```python
from build123d import *

# Parameters (mm, degrees)
SKETCH1_R           = 2
SKETCH1_R_2         = 6.5
BOSS_EXTRUDE1_DEPTH = 6


with BuildPart() as part:
    # Sketch1 → Boss-Extrude1 (new body)
    with BuildSketch(Plane(origin=(0, 0, 0), x_dir=(1, 0, 0), z_dir=(0, 1, 0))):
        with BuildLine():
            Line((-22.107690969, 10.5), (-42.5, 10.5))
            ThreePointArc((-42.5, 10.5), (-53, 0), (-42.5, -10.5))
            Line((-42.5, -10.5), (-22.107690969, -10.5))
            ThreePointArc((-22.107690969, -10.5), (-19.800295422, -11.06424462), (-18.013674085, -12.629629684))
            ThreePointArc((-18.013674085, -12.629629684), (7.2e-08, -22), (18.013674168, -12.629629566))
            ThreePointArc((18.013674168, -12.629629566), (19.800295486, -11.064244587), (22.107690969, -10.5))
            Line((22.107690969, -10.5), (42.5, -10.5))
            ThreePointArc((42.5, -10.5), (53, 0), (42.5, 10.5))
            Line((42.5, 10.5), (22.107690919, 10.5))
            ThreePointArc((22.107690919, 10.5), (19.800295464, 11.064244598), (18.013674168, 12.629629566))
            ThreePointArc((18.013674168, 12.629629566), (0, 22), (-18.013674168, 12.629629566))
            ThreePointArc((-18.013674168, 12.629629566), (-19.800295486, 11.064244587), (-22.107690969, 10.5))
        make_face()
        with Locations((17.989399487, 0.617661785)):
            Circle(SKETCH1_R, mode=Mode.SUBTRACT)
        with Locations((-42.5, 0)):
            Circle(SKETCH1_R_2, mode=Mode.SUBTRACT)
        with Locations((-18, 0)):
            Circle(SKETCH1_R, mode=Mode.SUBTRACT)
        with Locations((0, -18)):
            Circle(SKETCH1_R, mode=Mode.SUBTRACT)
        with Locations((0, 18)):
            Circle(SKETCH1_R, mode=Mode.SUBTRACT)
        with Locations((42.5, 0)):
            Circle(SKETCH1_R_2, mode=Mode.SUBTRACT)
    extrude(amount=BOSS_EXTRUDE1_DEPTH)


solid = part.part
```
Geometry: final body of the model. Coordinates: model frame, mm. A direction names the side the tool comes from. Coordinates: 2 decimals unless noted, no trailing zeros. Write each loop counter-clockwise with the first axis right and the second up, starting at its lowest first coordinate (ties: lowest second). Pieces come first, ordered by that corner, then holes. Notation, with made-up numbers: M 57,-4.75 L 61,-4.75 A23 ccw 61,27.25 Z; hole C 11,21.25 d5. An arc over 180 degrees is marked long. Answer as CSV lines item,"result". Start each with the question number.
Q1. Cut plane A-A on x = 0. Return the cut outline in (y, z).
Q2. Reachability of faces 1 (the flat face through (-32, 3, 10.5)), 2 (the cylindrical face through (0, 3, -22)), 3 (the flat face through (32, 3, 10.5)), 4 (the flat face through (-32, 3, -10.5)), 5 (the cylindrical face through (19.897, 2.958, -1.218)) from +Z, -Z, +X, -X, +Y, -Y: full face, straight path, thin tool, end or side. Return the list, or none.
Q3. Cut plane B-B on z = -5.5. Return the cut outline in (x, y).
Q4. Line query: line 1 (Z direction, x = 43, y = 3.65); line 2 (X direction, y = 2.85, z = 0); line 3 (X direction, y = 0.9, z = -19). Output: solid intervals per line, ascending. Write a range as from..to.
Q5. Mould query, pull axis X, two halves, no side actions, for faces 6 (the cylindrical face through (19.83, 2.96, -11.05)), 7 (the cylindrical face through (0, 3, 22)), 8 (the cylindrical face through (-49, 3, 0)). Classes: released by +X, released by -X, zero draft, split by the parting line, or undercut.
Q6. Cut plane D-D on z = -18. Return the cut outline in (x, y), then the cut area to 3 significant figures.
Q7. Pin query (flat end, axial travel): P1, Ø1, axis at x = 18, y = 2, coming from the +Z side; P2, Ø5, axis at x = -33, z = -12.5, coming from the -Y side; P3, Ø1.8, axis at x = -34.5, y = 2, coming from the +Z side. Return the tip coordinate at first contact, or that it passes through.
Q8. Cut plane C-C on y = 3. Return the cut outline in (x, z), then the cut area to 3 significant figures.
Findings below:
1,outline,"M 0,-22 L 6,-22 L 6,-20 L 0,-20 Z; M 0,-16 L 6,-16 L 6,16 L 0,16 Z; M 0,20 L 6,20 L 6,22 L 0,22 Z"
2,face 1,"+Z, -X, +Y, -Y"
2,face 2,"-Z, +Y, -Y"
2,face 3,"+Z, +X, +Y, -Y"
2,face 4,"-Z, -X, +Y, -Y"
2,face 5,"+Y, -Y"
3,outline,"M -51.44,0 L -45.96,0 L -45.96,6 L -51.44,6 Z; M -39.04,0 L 39.04,0 L 39.04,6 L -39.04,6 Z; M 45.96,0 L 51.44,0 L 51.44,6 L 45.96,6 Z"
4,line 1,"z = -10.49..-6.48, 6.48..10.49"
4,line 2,"x = -53..-49, -36..-20, -16..16.09, 19.89..36, 49..53"
4,line 3,"x = -11.09..-1.73, 1.73..11.09"
5,face 6,"released by +X"
5,face 7,"split by the parting line"
5,face 8,"undercut"
6,outline,"M -12.65,0 L -2,0 L -2,6 L -12.65,6 Z; M 2,0 L 12.65,0 L 12.65,6 L 2,6 Z"
6,area,"128 mm2"
7,P1,"stops at z = 13.33"
7,P2,"stops at y = 0"
7,P3,"stops at z = 10.5"
8,outline,"M -42.5,-10.5 L -22.11,-10.5 A5 cw -18.01,-12.63 A22 ccw 18.01,-12.63 A5 cw 22.11,-10.5 L 42.5,-10.5 A10.5 ccw 42.5,10.5 L 22.11,10.5 A5 cw 18.01,12.63 A22 ccw -18.01,12.63 A5 cw -22.11,10.5 L -42.5,10.5 A10.5 ccw Z; hole C -42.5,0 d13; hole C -18,0 d4; hole C 0,-18 d4; hole C 0,18 d4; hole C 17.99,-0.62 d4; hole C 42.5,0 d13"
8,area,"2,450 mm2"
